Can you work these out from the model? Positions are in its coordinate system, mm. A direction names the side the tool comes from. Give positions to 0.01 mm unless a question says otherwise; leave off trailing zeros. Order: outer loops, then holes, each group sorted by start corner. A loop starts at its lowest first (then second) coordinate and runs counter-clockwise, first axis right, second up. Notation, with made-up numbers: (86.25, 21.5) - (121.25, 21.5) arc R17 ccw to (121.25, 25.5) - close; hole circle Ø9 at (46.5, 37.25). An arc over 180 degrees is marked (long way). One line per question, with ' | ' between items.
```python
from build123d import *

# Parameters (mm, degrees)
F0_W     = 38.4
F0_H     = 28.4
F0_R     = 1.1
F0_R_2   = 4.1
F1_DEPTH = 1.5
F2_W     = 38.4
F2_H     = 1.5
F3_DEPTH = 22
F6_W     = 38.4
F6_H     = 14.2
F7_DEPTH = 25.001
F8_R     = 4
F8_R_2   = 1.1
F9_DEPTH = 1.5
F10_R    = 1


with BuildPart() as f1:
    # F0 (on Top) → F1 (new body)
    with BuildSketch(Plane.XY):
        Rectangle(F0_W, F0_H)
        with Locations((-16.2, -7.2)):
            Circle(F0_R, mode=Mode.SUBTRACT)
        with Locations((14.9, -7.2)):
            Circle(F0_R, mode=Mode.SUBTRACT)
        with Locations((-10, 0)):
            Circle(F0_R_2, mode=Mode.SUBTRACT)
        with Locations((-16.2, 7.2)):
            Circle(F0_R, mode=Mode.SUBTRACT)
        with BuildLine():
            ThreePointArc((-3, 4.8), (-1.5355339059, 8.3355339059), (2, 9.8))
            Line((2, 9.8), (11.7, 9.8))
            ThreePointArc((11.7, 9.8), (12.4071067812, 9.5071067812), (12.7, 8.8))
            Line((12.7, 8.8), (12.7, 5.5901699437))
            ThreePointArc((12.7, 5.5901699437), (12.7871290708, 5.1819216533), (13.0333333333, 4.8448139512))
            ThreePointArc((13.0333333333, 4.8448139512), (15.2, 0), (13.0333333333, -4.8448139512))
            ThreePointArc((13.0333333333, -4.8448139512), (12.7871290708, -5.1819216533), (12.7, -5.5901699437))
            Line((12.7, -5.5901699437), (12.7, -8.8))
            ThreePointArc((12.7, -8.8), (12.4071067812, -9.5071067812), (11.7, -9.8))
            Line((11.7, -9.8), (2, -9.8))
            ThreePointArc((2, -9.8), (-1.5355339059, -8.3355339059), (-3, -4.8))
            Line((-3, -4.8), (-3, 4.8))
        make_face(mode=Mode.SUBTRACT)
        with Locations((14.9, 7.2)):
            Circle(F0_R, mode=Mode.SUBTRACT)
    extrude(amount=F1_DEPTH)

    # F2 (on face) → F3 (join)
    with BuildSketch(Plane(origin=(0, 0, 0), x_dir=(1, 0, 0), z_dir=(0, 0, -1))):
        with Locations((0, 13.45)):
            Rectangle(F2_W, F2_H)
    extrude(amount=F3_DEPTH)

    # F5: F1 across plane


with BuildPart() as f1_1:
    add(f1.part)
    add(f1.part.mirror(Plane.XY.offset(-11)))

    # F6 (on face) → F7 (cut, through all)
    with BuildSketch(Plane(origin=(0, 0, -23.5), x_dir=(1, 0, 0), z_dir=(0, 0, -1))):
        with Locations((0, -7.1)):
            Rectangle(F6_W, F6_H)
    extrude(amount=-F7_DEPTH, mode=Mode.SUBTRACT)

    # F8 (on face) → F9 (cut, through all)
    with BuildSketch(Plane.XZ.offset(14.2)):
        with Locations((-10, -11)):
            Circle(F8_R)
        with Locations((-5.6, -6.6)):
            Circle(F8_R_2)
        with Locations((-10, -4.7774603256)):
            Circle(F8_R_2)
        with Locations((-14.4, -6.6)):
            Circle(F8_R_2)
        with Locations((-16.2225396744, -11)):
            Circle(F8_R_2)
        with Locations((-14.4, -15.4)):
            Circle(F8_R_2)
        with Locations((-10, -17.2225396744)):
            Circle(F8_R_2)
        with Locations((-5.6, -15.4)):
            Circle(F8_R_2)
        with Locations((-3.7774603256, -11)):
            Circle(F8_R_2)
        with Locations((10, -4.7774603256)):
            Circle(F8_R_2)
        with Locations((14.4, -15.4)):
            Circle(F8_R_2)
        with Locations((3.7774603256, -11)):
            Circle(F8_R_2)
        with Locations((16.2225396744, -11)):
            Circle(F8_R_2)
        with Locations((5.6, -15.4)):
            Circle(F8_R_2)
        with Locations((14.4, -6.6)):
            Circle(F8_R_2)
        with Locations((10, -17.2225396744)):
            Circle(F8_R_2)
        with Locations((10, -11)):
            Circle(F8_R)
        with Locations((5.6, -6.6)):
            Circle(F8_R_2)
    extrude(amount=-F9_DEPTH, mode=Mode.SUBTRACT)

    # F10
    f10_edges = [f1_1.edges().sort_by_distance(p)[0] for p in [
        (-19.2, 0, -22.75),
        (-19.2, 0, 0.75),
        (-5.9, 0, 0.75),
        (-14.1, 0, 0.75),
        (-5.9, 0, -22.75),
        (-14.1, 0, -22.75),
        (-3, 0, -22.75),
        (15.2, 0, -22.75),
        (15.2, 0, 0.75),
        (19.2, 0, -22.75),
        (19.2, 0, 0.75),
        (-3, 0, 0.75),
    ]]
    fillet(f10_edges, radius=F10_R)


solid = f1_1.part
```
(1) Imagine slicing it at C-C (z = -6.6). List the corners of the cut face in (x, y) for me.
Answer below:
outline: (-19.2, -14.2) - (-15.5, -14.2) - (-15.5, -12.7) - (-19.2, -12.7) - close; (-13.3, -14.2) - (-6.7, -14.2) - (-6.7, -12.7) - (-13.3, -12.7) - close; (-4.5, -14.2) - (4.5, -14.2) - (4.5, -12.7) - (-4.5, -12.7) - close; (6.7, -14.2) - (13.3, -14.2) - (13.3, -12.7) - (6.7, -12.7) - close; (15.5, -14.2) - (19.2, -14.2) - (19.2, -12.7) - (15.5, -12.7) - close
(2) Imagine slicing it at A-A (y = -10.75). List the corners of the cut face in (x, z) for me, and give its area (3 significant figures).
Answer below:
outline: (-19.2, -23.5) - (19.2, -23.5) - (19.2, -22) - (-19.2, -22) - close; (-19.2, 0) - (19.2, 0) - (19.2, 1.5) - (-19.2, 1.5) - close | area: 115 mm^2
(3) If we mould it in two halves opening along Y, with no side actions, what happens to faces 1 (the face through (15.916, -7.621, 0.74)), 2 (the face through (-8.984, -13.46, -17.644)), 3 (the face through (-15.184, -7.621, 0.74)), 4 (the face through (7, -9.8, -23))? For each: released by +Y, released by -Y, zero draft, split by the parting line, or undercut.
Answer below:
face 1: undercut | face 2: zero draft | face 3: undercut | face 4: released by +Y
(4) If I drill on line 1 (Z direction, x = -10, y = -13.7); line 2 (Z direction, x = -2, y = -10.5); line 3 (Z direction, x = -5.6, y = -13.25), over which ranges is the centre line in solid material (lowest first)?
Answer below:
line 1: -23.5 to -18.32, -16.12 to -15, -7 to -5.88, -3.68 to 1.5 | line 2: -23.5 to -22, 0 to 1.5 | line 3: -23.5 to -16.5, -14.3 to -7.7, -5.5 to 1.5
(5) On a 3-axis mill with a long thin cutter (end or side, diameter ignored), from which of +Z, -Z, +X, -X, +Y, -Y can I reach the whole of each face in a straight line? I mean faces 5 (the face through (-4.584, -13.46, -7.021)), 6 (the face through (15.47, -0.25, -22.74)). Say none if no direction works.
Answer below:
face 5: +Y, -Y | face 6: +Z, -Z, +Y
(6) Imagine slicing it at D-D (z = -13.5). List the corners of the cut face in (x, y) for me.
Answer below:
outline: (-19.2, -14.2) - (-13.12, -14.2) - (-13.12, -12.7) - (-19.2, -12.7) - close; (-6.88, -14.2) - (6.88, -14.2) - (6.88, -12.7) - (-6.88, -12.7) - close; (13.12, -14.2) - (19.2, -14.2) - (19.2, -12.7) - (13.12, -12.7) - close
(7) Will this pin go through, and if not, where does the flat tip stop? pin 1 (1.5 mm diameter, centred on x = -12, z = -4.5, fed in from +Y).
Answer below:
pin 1: y = -12.7
(8) Imagine slicing it at B-B (x = -10). List the corners of the cut face in (y, z) for me.
Answer below:
outline: (-14.2, -23.5) - (-4.1, -23.5) - (-4.1, -22) - (-12.7, -22) - (-12.7, -18.32) - (-14.2, -18.32) - close; (-14.2, -16.12) - (-12.7, -16.12) - (-12.7, -15) - (-14.2, -15) - close; (-14.2, -7) - (-12.7, -7) - (-12.7, -5.88) - (-14.2, -5.88) - close; (-14.2, -3.68) - (-12.7, -3.68) - (-12.7, 0) - (-4.1, 0) - (-4.1, 1.5) - (-14.2, 1.5) - close
